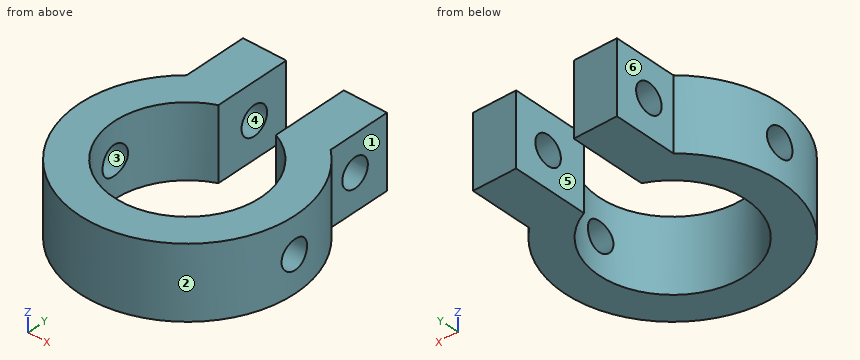
```python
from build123d import *

# Parameters (mm, degrees)
CYLINDER003_R     = 2
CYLINDER003_DEPTH = 40
CYLINDER002_R     = 2
CYLINDER002_DEPTH = 40
CYLINDER001_R     = 10.2
CYLINDER001_DEPTH = 10
BOX001_W          = 8
BOX001_H          = 15
BOX001_DEPTH      = 10
BOX_W             = 20
BOX_H             = 10
BOX_DEPTH         = 10
CYLINDER_R        = 15
CYLINDER_DEPTH    = 10


with BuildPart() as cylinder003:
    # Cylinder003 → Cylinder003 (new body)
    with BuildSketch(Plane(origin=(-20, 15, 5), x_dir=(0, 0, -1), z_dir=(1, 0, 0))):
        Circle(CYLINDER003_R)
    extrude(amount=CYLINDER003_DEPTH)


with BuildPart() as cylinder002:
    # Cylinder002 → Cylinder002 (new body)
    with BuildSketch(Plane(origin=(-20, 0, 5), x_dir=(0, 0, -1), z_dir=(1, 0, 0))):
        Circle(CYLINDER002_R)
    extrude(amount=CYLINDER002_DEPTH)


with BuildPart() as cylinder001:
    # Cylinder001 → Cylinder001 (new body)
    with BuildSketch(Plane.XY):
        Circle(CYLINDER001_R)
    extrude(amount=CYLINDER001_DEPTH)


with BuildPart() as negative_fusion:
    # Box001 → Box001 (new body)
    with BuildSketch(Plane(origin=(-4, 5, 0), x_dir=(1, 0, 0), z_dir=(0, 0, 1))):
        with Locations((4, 7.5)):
            Rectangle(BOX001_W, BOX001_H)
    extrude(amount=BOX001_DEPTH)

    # Fusion001: union Cylinder003, Cylinder002, Cylinder001
    add(cylinder003.part)
    add(cylinder002.part)
    add(cylinder001.part)


with BuildPart() as cube:
    # Box → Box (new body)
    with BuildSketch(Plane(origin=(-10, 10, 0), x_dir=(1, 0, 0), z_dir=(0, 0, 1))):
        with Locations((10, 5)):
            Rectangle(BOX_W, BOX_H)
    extrude(amount=BOX_DEPTH)


with BuildPart() as cut:
    # Cylinder → Cylinder (new body)
    with BuildSketch(Plane.XY):
        Circle(CYLINDER_R)
    extrude(amount=CYLINDER_DEPTH)

    # Fusion: union Cube
    add(cube.part)

    # Cut: cut Negative Fusion
    add(negative_fusion.part, mode=Mode.SUBTRACT)


solid = cut.part
```
The model under review builds one solid part; all positions refer to its coordinate system, in mm. Face numbers are marked on the shaded views. A direction names the side the tool comes from. Round coordinates to 2 decimals unless told otherwise and drop trailing zeros. Write each loop counter-clockwise with the first axis right and the second up, starting at its lowest first coordinate (ties: lowest second). Pieces come first, ordered by that corner, then holes.
(1) Wall thickness on L1, parallel to Z at x = -12.1, y = 0; L2, parallel to Y at x = -5, z = 4; L3, parallel to X at y = 13, z = 1: over which ranges is each line inside the solid? List them lowest first.
(2) Mouldability with a two-part tool opening along Y and no side actions: class the marked faces 1, 2 and 3 as +Y half, -Y half, draft (parallel to the pull), parting line (faces both ways), or undercut.
(3) We need section A-A on y = 0. Give the boundary of the cut face in (x, z), and give its area (3 significant figures).
(4) We need section B-B on x = 6.5. Give the boundary of the cut face in (y, z).
(5) Insertion check: pin 1 (2 mm diameter, centred on x = -11, z = 4.5, fed in from -Y); pin 2 (3 mm diameter, centred on y = 14, z = 3.5, fed in from -X); pin 3 (6 mm diameter, centred on x = 9, z = 8, fed in from -Y). Each pin has a flat end and moves straight along its axis. Give the tip position at first contact, or say it passes through.
(6) We need section D-D on z = 6.25. Give the boundary of the cut face in (x, y), and give its area (3 significant figures).
(7) We need section C-C on y = 12. Give the boundary of the cut face in (x, z), and give its area (3 significant figures).
(8) Machinability: for the marked faces 4, 5 and 6, which of the approach directions +Z, -Z, +X, -X, +Y, -Y give a long, thin tool a straight path to every point of the face, cutting with its end or side? Answer none if there is none.
Findings below:
1. L1: z = 0 to 3, 7 to 10
1. L2: y = -14.14 to -8.89, 8.89 to 13.27, 16.73 to 20
1. L3: x = -10 to -4, 4 to 10
2. face 1: draft
2. face 2: parting line
2. face 3: undercut
3. outline: (-15, 0) - (-10.2, 0) - (-10.2, 3) - (-15, 3) - close; (-15, 7) - (-10.2, 7) - (-10.2, 10) - (-15, 10) - close; (10.2, 0) - (15, 0) - (15, 3) - (10.2, 3) - close; (10.2, 7) - (15, 7) - (15, 10) - (10.2, 10) - close
3. area: 57.6 mm2
4. outline: (-13.52, 0) - (-7.86, 0) - (-7.86, 10) - (-13.52, 10) - close; (7.86, 0) - (20, 0) - (20, 10) - (7.86, 10) - close; hole circle Ø4 at (15, 5)
5. pin 1: stops at y = -11.18
5. pin 2: stops at x = -10
5. pin 3: stops at y = -13.75
6. outline: (-14.92, -1.56) arc R15 ccw to (14.92, -1.56) - (10.08, -1.56) arc R10.2 cw to (-10.08, -1.56) - close; (-14.92, 1.56) - (-10.08, 1.56) arc R10.2 cw to (-4, 9.38) - (-4, 13.44) - (-10, 13.44) - (-10, 11.18) arc R15 ccw to start; (-10, 16.56) - (-4, 16.56) - (-4, 20) - (-10, 20) - close; (4, 9.38) arc R10.2 cw to (10.08, 1.56) - (14.92, 1.56) arc R15 ccw to (10, 11.18) - (10, 13.44) - (4, 13.44) - close; (4, 16.56) - (10, 16.56) - (10, 20) - (4, 20) - close
6. area: 356 mm2
7. outline: (-10, 0) - (-4, 0) - (-4, 10) - (-10, 10) - close; (4, 0) - (10, 0) - (10, 10) - (4, 10) - close
7. area: 120 mm2
8. face 4: +X, -X
8. face 5: +Z, -Z, +Y
8. face 6: +Z, -Z, -X, +Y
